```python
from build123d import *

# Parameters (mm, degrees)
SKETCH1_R           = 15.591175954
BOSS_EXTRUDE1_DEPTH = 71
BOSS_EXTRUDE2_START = 1.25
SKETCH2_R           = 15.591175954
SKETCH2_W           = 17.8
SKETCH2_H           = 1.65
BOSS_EXTRUDE2_DEPTH = 1.25
BOSS_EXTRUDE3_START = 4
SKETCH3_R           = 15.591175954
BOSS_EXTRUDE3_DEPTH = 4
CUT_EXTRUDE4_START  = -11.5
SKETCH16_R          = 0.75
CUT_EXTRUDE4_DEPTH  = 11.5
BOSS_EXTRUDE8_START = 10
SKETCH18_R          = 15.591175954
SKETCH18_R_2        = 13.095738675
BOSS_EXTRUDE8_DEPTH = 10
FILLET3_START       = -12.2500001
FILLET3_OUTLINE_R   = 13.095738675
FILLET3_OUTLINE_R_2 = 0.75
FILLET3_DEPTH       = 7.0000001
FILLET3_START_2     = -11
FILLET3_3_DEPTH     = 5.75


with BuildPart() as part:
    # Sketch1 → Boss-Extrude1 (new body)
    with BuildSketch(Plane(origin=(0, 0, 0), x_dir=(1, 0, 0), z_dir=(0, 1, 0))):
        with Locations(Location((0, 0, 0), (0, 0, 270))):
            Circle(SKETCH1_R)
        with BuildLine():
            Line((8.375, -6.964282891), (9.075, -6.964282891))
            Line((9.075, -6.964282891), (9.075, -8.614282891))
            Line((9.075, -8.614282891), (8.375, -8.614282891))
            Line((8.375, -8.614282891), (8.375, -9.610929808))
            ThreePointArc((8.375, -9.610929808), (0, -12.747964417), (-8.375, -9.610929808))
            Line((-8.375, -9.610929808), (-8.375, -8.614282891))
            Line((-8.375, -8.614282891), (-8.725, -8.614282891))
            Line((-8.725, -8.614282891), (-8.725, -6.964282891))
            Line((-8.725, -6.964282891), (-8.375, -6.964282891))
            Line((-8.375, -6.964282891), (-8.375, -6.204282891))
            Line((-8.375, -6.204282891), (-8.375, 9.645717109))
            ThreePointArc((-8.375, 9.645717109), (-7.386485387, 12.032202496), (-5, 13.020717109))
            Line((-5, 13.020717109), (5, 13.020717109))
            ThreePointArc((5, 13.020717109), (7.386485387, 12.032202496), (8.375, 9.645717109))
            Line((8.375, 9.645717109), (8.375, -6.204282891))
            Line((8.375, -6.204282891), (8.375, -6.964282891))
        make_face(mode=Mode.SUBTRACT)
    extrude(amount=BOSS_EXTRUDE1_DEPTH)

    # Sketch2 → Boss-Extrude2 (add)
    with BuildSketch(Plane.XZ.offset(BOSS_EXTRUDE2_START)):
        with Locations(Location((0, 0, 0), (0, 0, 270))):
            Circle(SKETCH2_R)
        with Locations((0.175, 7.789282891)):
            Rectangle(SKETCH2_W, SKETCH2_H, mode=Mode.SUBTRACT)
    extrude(amount=-BOSS_EXTRUDE2_DEPTH)

    # Sketch3 → Boss-Extrude3 (add)
    with BuildSketch(Plane.XZ.offset(1.25).offset(BOSS_EXTRUDE3_START)):
        with Locations(Location((0, 0, 0), (0, 0, 270))):
            Circle(SKETCH3_R)
    extrude(amount=-BOSS_EXTRUDE3_DEPTH)

    # Sketch16 → Cut-Extrude4 (cut)
    with BuildSketch(Plane(origin=(0, 0, 0), x_dir=(1, 0, 0), z_dir=(0, 1, 0)).offset(CUT_EXTRUDE4_START)):
        with BuildLine():
            Line((-3.75, -9.901070776), (-3, -9.901070776))
            Line((-3, -9.901070776), (-2.25, -9.901070776))
            ThreePointArc((-2.25, -9.901070776), (-3, -9.151070776), (-3.75, -9.901070776))
        make_face()
        with BuildLine():
            Line((-2.25, -9.901070776), (-3, -9.901070776))
            Line((-3, -9.901070776), (-3.75, -9.901070776))
            ThreePointArc((-3.75, -9.901070776), (-3, -10.651070776), (-2.25, -9.901070776))
        make_face()
        with BuildLine():
            ThreePointArc((6.75, -9.901070776), (6, -9.151070776), (5.25, -9.901070776))
            ThreePointArc((5.25, -9.901070776), (6, -10.651070776), (6.75, -9.901070776))
        make_face()
        with BuildLine():
            ThreePointArc((3.75, -9.901070776), (3, -9.151070776), (2.25, -9.901070776))
            Line((2.25, -9.901070776), (3, -9.901070776))
            Line((3, -9.901070776), (3.75, -9.901070776))
        make_face()
        with BuildLine():
            Line((3, -9.901070776), (2.25, -9.901070776))
            ThreePointArc((2.25, -9.901070776), (3, -10.651070776), (3.75, -9.901070776))
            Line((3.75, -9.901070776), (3, -9.901070776))
        make_face()
        with BuildLine():
            ThreePointArc((0.75, -9.901070776), (0, -9.151070776), (-0.75, -9.901070776))
            Line((-0.75, -9.901070776), (0, -9.901070776))
            Line((0, -9.901070776), (0.75, -9.901070776))
        make_face()
        with BuildLine():
            Line((0, -9.901070776), (-0.75, -9.901070776))
            ThreePointArc((-0.75, -9.901070776), (0, -10.651070776), (0.75, -9.901070776))
            Line((0.75, -9.901070776), (0, -9.901070776))
        make_face()
        with Locations(Location((-6, -9.901070776, 0), (0, 0, 270))):
            Circle(SKETCH16_R)
        with BuildLine():
            ThreePointArc((5.289192257, -11.598924176), (4.550417773, -10.824582592), (3.789595018, -11.577272013))
            ThreePointArc((3.789595018, -11.577272013), (3.846450326, -11.860961254), (4.006459728, -12.102019552))
            ThreePointArc((4.006459728, -12.102019552), (4.654628095, -11.867815051), (5.289192257, -11.598924176))
        make_face()
        with BuildLine():
            ThreePointArc((2.290136401, -11.577272013), (1.540136401, -10.827272013), (0.790136401, -11.577272013))
            Line((0.790136401, -11.577272013), (1.540136401, -11.577272013))
            Line((1.540136401, -11.577272013), (2.290136401, -11.577272013))
        make_face()
        with BuildLine():
            Line((1.540136401, -11.577272013), (0.790136401, -11.577272013))
            ThreePointArc((0.790136401, -11.577272013), (1.540136401, -12.327272013), (2.290136401, -11.577272013))
            Line((2.290136401, -11.577272013), (1.540136401, -11.577272013))
        make_face()
        with BuildLine():
            ThreePointArc((-0.707561207, -11.577133163), (-2.207561203, -11.577063737), (-0.707561219, -11.577272013))
            ThreePointArc((-0.707561219, -11.577272013), (-0.70756121, -11.577202588), (-0.707561207, -11.577133163))
        make_face()
        with BuildLine():
            ThreePointArc((-5.205190023, -11.636863564), (-4.580517042, -11.896615502), (-3.942943702, -12.122862358))
            ThreePointArc((-3.942943702, -12.122862358), (-4.188076003, -10.877359358), (-5.205190023, -11.636863564))
        make_face()
    extrude(amount=CUT_EXTRUDE4_DEPTH, mode=Mode.SUBTRACT)

    # Sketch18 → Boss-Extrude8 (add)
    with BuildSketch(Plane.XZ.offset(5.25).offset(BOSS_EXTRUDE8_START)):
        with Locations(Location((0, 0, 0), (0, 0, 270))):
            Circle(SKETCH18_R)
        with Locations(Location((0, 0, 0), (0, 0, 270))):
            Circle(SKETCH18_R_2, mode=Mode.SUBTRACT)
    extrude(amount=-BOSS_EXTRUDE8_DEPTH)

    # Fillet3: read off the stored shape, not the designer's step
    # Fillet3 outline → Fillet3 (add)
    with BuildSketch(Plane(origin=(0, 0, 0), x_dir=(1, 0, 0), z_dir=(0, 1, 0)).offset(FILLET3_START)):
        Circle(FILLET3_OUTLINE_R)
        with Locations((-6, -9.901070776)):
            Circle(FILLET3_OUTLINE_R_2, mode=Mode.SUBTRACT)
        with Locations((-1.457561207, -11.577133163)):
            Circle(FILLET3_OUTLINE_R_2, mode=Mode.SUBTRACT)
        with Locations((-3, -9.901070776)):
            Circle(FILLET3_OUTLINE_R_2, mode=Mode.SUBTRACT)
        with Locations((1.540136401, -11.577272013)):
            Circle(FILLET3_OUTLINE_R_2, mode=Mode.SUBTRACT)
        with Locations((0, -9.901070776)):
            Circle(FILLET3_OUTLINE_R_2, mode=Mode.SUBTRACT)
        with Locations((3, -9.901070776)):
            Circle(FILLET3_OUTLINE_R_2, mode=Mode.SUBTRACT)
        with Locations((6, -9.901070776)):
            Circle(FILLET3_OUTLINE_R_2, mode=Mode.SUBTRACT)
    extrude(amount=FILLET3_DEPTH)

    # Fillet3 2 outline → Fillet3 2 (revolve, cut)
    with BuildSketch(Plane.XY):
        with BuildLine():
            Line((6.095738675, -5.25), (0, -5.25))
            Line((0, -5.25), (0, -12.25))
            Line((0, -12.25), (13.095738675, -12.25))
            ThreePointArc((13.095738675, -12.25), (11.045486143, -7.300252532), (6.095738675, -5.25))
        make_face()
    revolve(axis=Axis((0, 0, 0), (0, 1, 0)), mode=Mode.SUBTRACT)

    # Fillet3 3 outline → Fillet3 3 (cut)
    with BuildSketch(Plane(origin=(0, 0, 0), x_dir=(1, 0, 0), z_dir=(0, 1, 0)).offset(FILLET3_START_2)):
        with BuildLine():
            ThreePointArc((4.006459728, -12.102019552), (4.654628094, -11.867815051), (5.289192257, -11.598924176))
            ThreePointArc((5.289192257, -11.598924176), (4.265744538, -10.876286186), (4.006459728, -12.102019552))
        make_face()
        with BuildLine():
            ThreePointArc((-5.205190023, -11.636863564), (-4.580517042, -11.896615502), (-3.942943702, -12.122862358))
            ThreePointArc((-3.942943702, -12.122862358), (-4.188076003, -10.877359358), (-5.205190023, -11.636863564))
        make_face()
    extrude(amount=FILLET3_3_DEPTH, mode=Mode.SUBTRACT)


solid = part.part
```
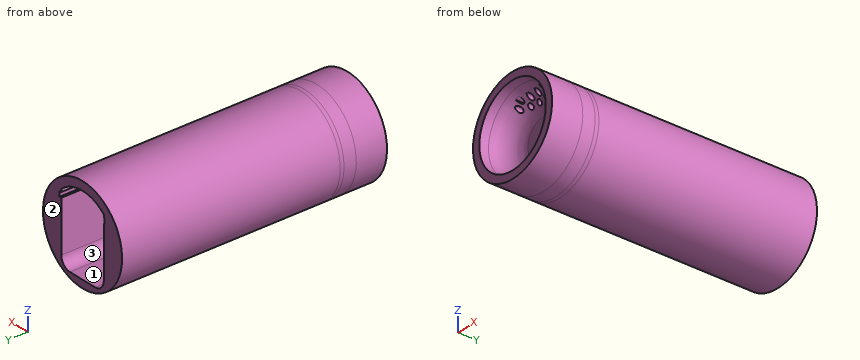
Could you check a few things on this model? Use its own coordinates, in mm. Face numbers are marked on the shaded views. Give positions to 0.01 mm unless a question says otherwise; leave off trailing zeros. Loops run counter-clockwise (first coordinate to the right, second up) from the corner with the lowest first, then second, coordinate; pieces in that order, holes last. Notation, with made-up numbers: (86.25, 86.25) - (131.25, 86.25) arc R22 cw to (131.25, 99.25) - close; hole circle Ø4 at (9.25, 54). An arc over 180 degrees is marked (long way). Answer in a Markdown table with one row per item. Add a question column.
Q1. We'd pull the mould along Z, two halves only. Please class the marked faces 1, 2 and 3: +Z half, -Z half, draft (parallel to the pull), parting line (faces both ways), or undercut.
Q2. Please list where these lines run through material, in increasing order: L1, parallel to Y at x = -3.5, z = -3.5; L2, parallel to X at y = 5.5, z = 6 (3 decimals); L3, parallel to Z at x = -7, y = 21. Write a range as from..to.
Q3. For pin 1 (2 mm diameter, centred on x = 0.5, z = 9.5, fed in from +Y); pin 2 (10 mm diameter, centred on x = 0.5, z = -2, fed in from -Y); pin 3 (1.3 mm diameter, centred on x = -1.46, z = 11.58, fed in from -Y); pin 4 (6 mm diameter, centred on x = 3.5, y = 20.5, fed in from -Z), each with a flat end and sliding along its axis, tell me the tip position at first contact or that it passes through.
Q4. If we section it at A-A (y = 39): List the corners of the cut face in (x, z) for me (3 decimals), plus the area to 3 significant figures.
The answers:
| question | item | result |
|---|---|---|
| 1 | face 1 | undercut |
| 1 | face 2 | draft |
| 1 | face 3 | undercut |
| 2 | L1 | y = -5.25..0 |
| 2 | L2 | x = -14.39..-8.375, 8.375..14.39 |
| 2 | L3 | z = -13.93..-12.36, 10.65..13.93 |
| 3 | pin 1 | stops at y = 0 |
| 3 | pin 2 | stops at y = -5.32 |
| 3 | pin 3 | passes through |
| 3 | pin 4 | stops at z = -15.58 |
| 4 | outline | circle Ø31.182 at (0, 0); hole (-8.725, 6.964) - (-8.375, 6.964) - (-8.375, -9.646) arc R3.375 ccw to (-5, -13.021) - (5, -13.021) arc R3.375 ccw to (8.375, -9.646) - (8.375, 6.964) - (9.075, 6.964) - (9.075, 8.614) - (8.375, 8.614) - (8.375, 9.611) arc R12.748 ccw to (-8.375, 9.611) - (-8.375, 8.614) - (-8.725, 8.614) - close |
| 4 | area | 352 mm^2 |
